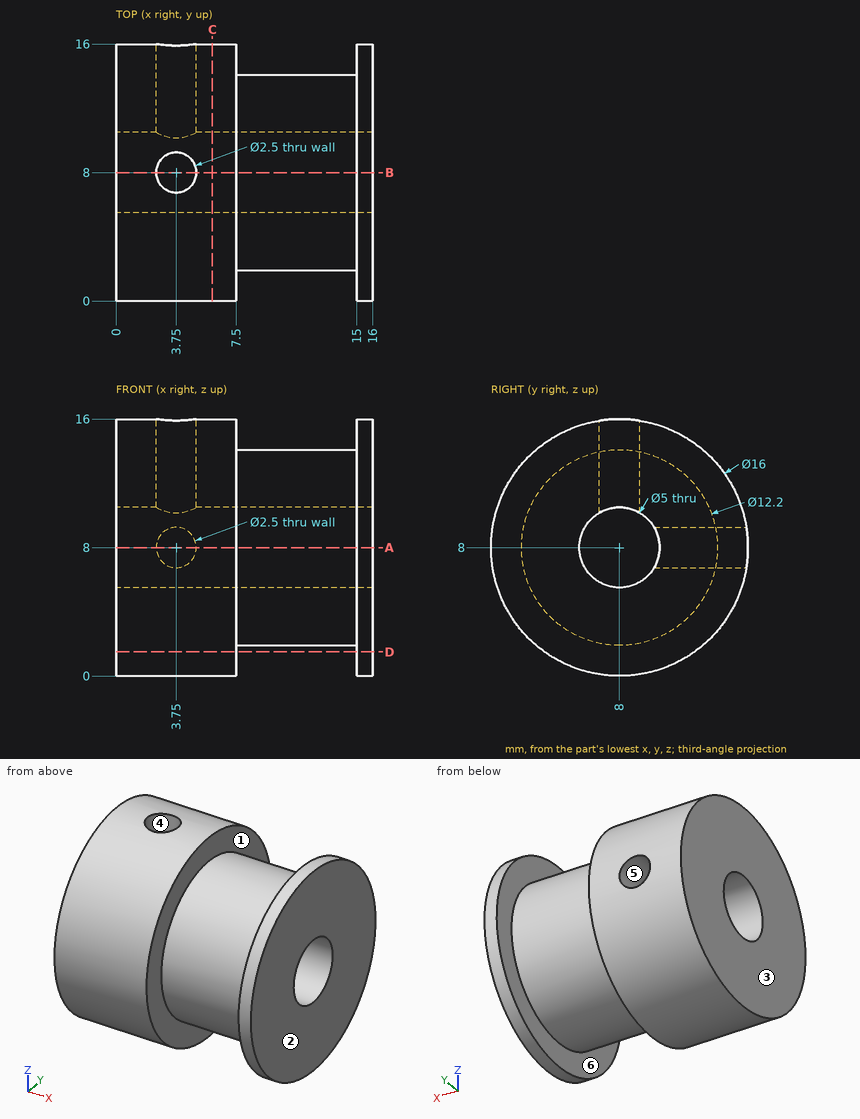
Job drawing, mm, ordinate dimensions from the low corner. One solid piece. A direction names the side the tool comes from. Round coordinates to 2 decimals unless told otherwise and drop trailing zeros. Loops run counter-clockwise (first coordinate to the right, second up) from the corner with the lowest first, then second, coordinate; pieces in that order, holes last. Notation, with made-up numbers: (83, 64.25) -> (91, 64.25) arc R14 ccw to (91, 86.25) -> close; hole circle Ø7 at (71, -25). An arc over 180 degrees is marked (long way). Use a Markdown table: item, result.
1) Probe line 1 (Y direction, x = 11, z = 8); line 2 (X direction, y = 1, z = 6); line 3 (Y direction, x = 8, z = 6.5). List the from-to ranges inside material, lowest first. Write a range as [from, to].
The answers:
| item | result |
|---|---|
| line 1 | y = [1.9, 5.5], [10.5, 14.1] |
| line 2 | x = [0, 7.5], [15, 16] |
| line 3 | y = [2.09, 6], [10, 13.91] |
2) Drop flat-ended pins along their axis: pin 1 Ø1.5 at (x, z) = (2.5, 14.5) entering from +Y; pin 2 Ø6 at (x, y) = (5, 2.5) entering from +Z; pin 3 Ø4 at (x, z) = (10, 6.5) entering from -Y. Give the stop position or say it passes through.
The answers:
| item | result |
|---|---|
| pin 1 | stops at y = 13.56 |
| pin 2 | stops at z = 15.6 |
| pin 3 | stops at y = 1.9 |
3) Cut at C-C, the plane x = 6. List the corners of the cut face in (y, z).
The answers:
| item | result |
|---|---|
| outline | circle Ø16 at (8, 8); hole circle Ø5 at (8, 8) |
4) Tool access for the marked faces 4, 5 and 6: list every direction of +Z, -Z, +X, -X, +Y, -Y with a clear straight run to the whole face (end or side of a thin tool).
The answers:
| item | result |
|---|---|
| face 4 | +Z |
| face 5 | +Y |
| face 6 | none |
5) Pull direction X, two halves, no side cores. Call the marked faces 1, 2 and 3: pulls with the +X half, pulls with the -X half, needs draft (parallel to the pull), parting line crosses it, or undercut.
The answers:
| item | result |
|---|---|
| face 1 | undercut |
| face 2 | pulls with the +X half |
| face 3 | pulls with the -X half |
6) Cut at A-A, the plane z = 8. List the corners of the cut face in (x, y), and give its area (3 significant figures).
The answers:
| item | result |
|---|---|
| outline | (0, 0) -> (7.5, 0) -> (7.5, 1.9) -> (15, 1.9) -> (15, 0) -> (16, 0) -> (16, 5.5) -> (0, 5.5) -> close; (0, 10.5) -> (2.5, 10.5) -> (2.5, 16) -> (0, 16) -> close; (5, 10.5) -> (16, 10.5) -> (16, 16) -> (15, 16) -> (15, 14.1) -> (7.5, 14.1) -> (7.5, 16) -> (5, 16) -> close |
| area | 134 mm2 |
7) Cut at D-D, the plane z = 1.5. List the corners of the cut face in (x, y).
The answers:
| item | result |
|---|---|
| outline | (0, 3.34) -> (7.5, 3.34) -> (7.5, 12.66) -> (0, 12.66) -> close; (15, 3.34) -> (16, 3.34) -> (16, 12.66) -> (15, 12.66) -> close |
